CAD build for the part. Positions are in the model's coordinates, mm. Give positions to 0.01 mm unless a question says otherwise; leave off trailing zeros. Write each loop counter-clockwise with the first axis right and the second up, starting at its lowest first coordinate (ties: lowest second). Pieces come first, ordered by that corner, then holes. Notation, with made-up numbers: (49.25, 2) - (69.25, 2) arc R29 ccw to (69.25, 34) - close; hole circle Ø10 at (89.5, 73). An arc over 180 degrees is marked (long way). Answer as a JSON object with one key per item and string values.
from build123d import *

# Parameters (mm, degrees)
F1_DEPTH = 1
F3_D     = 3.048
F3_DEPTH = 12.7
F3_TIP   = 0.9157115834


# Not quite as in the source:
# - a feature names something its author has since deleted; it is built from what else it names


with BuildPart() as f1:
    # F0 (on Top) → F1 (new body)
    with BuildSketch(Plane.XY):
        Polygon((127, 56.1535057819), (-127, 56.1535057819), (-127, 11.7035057819), (-127, -64.4964942181), (19.05, -64.4964942181), (19.05, 11.7035057819), (127, 11.7035057819), align=None)
    extrude(amount=F1_DEPTH)

    # F3
    with Locations(Plane.XY.offset(1)):
        with Locations((-120.65, 49.8035057819), (-120.65, -4.1714942181), (-120.65, -58.1464942181), (12.7, -58.1464942181), (12.7, -4.1714942181), (120.65, 49.8035057819)):
            Hole(F3_D / 2, depth=F3_DEPTH)
            with Locations((0, 0, -(F3_DEPTH + F3_TIP / 2))):  # 118° drill point
                Cone(0, F3_D / 2, F3_TIP, mode=Mode.SUBTRACT)


solid = f1.part
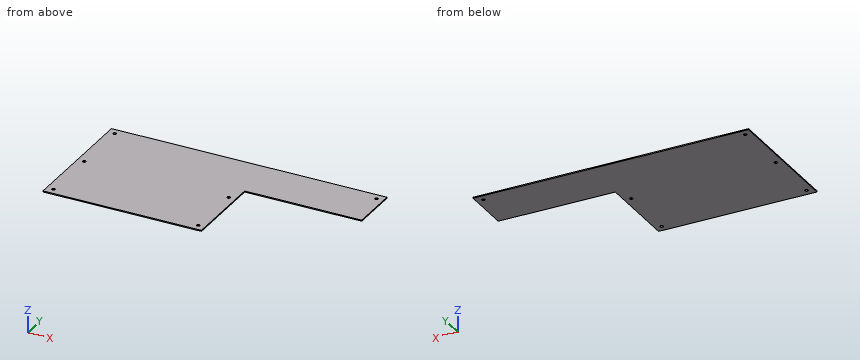
(1) Saw through at A-A, the plane z = 0.7. Give the cut face in (x, y), and give its area (3 significant figures).
Answer key:
{"outline": "(-127, -64.5) - (19.05, -64.5) - (19.05, 11.7) - (127, 11.7) - (127, 56.15) - (-127, 56.15) - close; hole circle Ø3.05 at (-120.65, -58.15); hole circle Ø3.05 at (-120.65, -4.17); hole circle Ø3.05 at (-120.65, 49.8); hole circle Ø3.05 at (12.7, -58.15); hole circle Ø3.05 at (12.7, -4.17); hole circle Ø3.05 at (120.65, 49.8)", "area": "22,400 mm²"}
(2) Probe L1, parallel to Y at x = 12.7, z = 0.4; L2, parallel to Y at x = -120.65, z = 0.3; L3, parallel to Y at x = 120.65, z = 0.45. List the from-to ranges inside material, lowest first. Write a range as [from, to].
Answer key:
{"L1": "y = [-64.5, -59.67], [-56.62, -5.7], [-2.65, 56.15]", "L2": "y = [-64.5, -59.67], [-56.62, -5.7], [-2.65, 48.28], [51.33, 56.15]", "L3": "y = [11.7, 48.28], [51.33, 56.15]"}
(3) Flat gauge pin, fed straight in: P1, Ø0.5, axis at y = -25, z = 0.5, coming from the +X side. Where does the tip first touch, or does it go through?
Answer key:
{"P1": "stops at x = 19.05"}
(4) Saw through at C-C, the plane x = 41.5. Give the cut face in (y, z), and give its area (4 significant figures).
Answer key:
{"outline": "(11.7, 0) - (56.15, 0) - (56.15, 1) - (11.7, 1) - close", "area": "44.45 mm²"}
(5) Saw through at B-B, the plane y = 8. Give the cut face in (x, z).
Answer key:
{"outline": "(-127, 0) - (19.05, 0) - (19.05, 1) - (-127, 1) - close"}
